from build123d import *

# Parameters (mm, degrees)
SCHIZZO1_W                   = 42.3
SCHIZZO1_H                   = 42.3
ESTRUSIONE_ESTRUSIONE1_DEPTH = 48
SMUSSO1_SIZE                 = 5
SCHIZZO2_R                   = 2.5
ESTRUSIONE_ESTRUSIONE2_DEPTH = 26
SCHIZZO3_W                   = 2.3
SCHIZZO3_H                   = 15
ESTRUSIONE_ESTRUSIONE3_DEPTH = 5
SCHIZZO4_R                   = 1.5
TAGLIO_ESTRUSIONE1_DEPTH     = 5


with BuildPart() as part:
    # Schizzo1 → Estrusione-Estrusione1 (new body)
    with BuildSketch(Plane.XY):
        Rectangle(SCHIZZO1_W, SCHIZZO1_H)
    extrude(amount=ESTRUSIONE_ESTRUSIONE1_DEPTH)

    # Smusso1
    smusso1_edges = [part.edges().sort_by_distance(p)[0] for p in [
        (21.15, -21.15, 24),
        (-21.15, -21.15, 24),
        (-21.15, 21.15, 24),
        (21.15, 21.15, 24),
    ]]
    chamfer(smusso1_edges, length=SMUSSO1_SIZE)

    # Schizzo2 → Estrusione-Estrusione2 (add)
    with BuildSketch(Plane.XY.offset(48)):
        Circle(SCHIZZO2_R)
    extrude(amount=ESTRUSIONE_ESTRUSIONE2_DEPTH)

    # Schizzo3 → Estrusione-Estrusione3 (add)
    with BuildSketch(Plane(origin=(0, 0, 0), x_dir=(-1, 0, 0), z_dir=(0, 0, -1))):
        with Locations((0, -28.65)):
            Rectangle(SCHIZZO3_W, SCHIZZO3_H)
    extrude(amount=-ESTRUSIONE_ESTRUSIONE3_DEPTH)

    # Schizzo4 → Taglio-Estrusione1 (cut)
    with BuildSketch(Plane.XY.offset(48)):
        with Locations((-15.5, 15.5)):
            Circle(SCHIZZO4_R)
        with Locations((-15.5, -15.5)):
            Circle(SCHIZZO4_R)
        with Locations((15.5, -15.5)):
            Circle(SCHIZZO4_R)
        with Locations((15.5, 15.5)):
            Circle(SCHIZZO4_R)
    extrude(amount=-TAGLIO_ESTRUSIONE1_DEPTH, mode=Mode.SUBTRACT)


solid = part.part
Verification items for the finished model (mm, model axes). A direction names the side the tool comes from. Give positions to 0.01 mm unless a question says otherwise; leave off trailing zeros. Loops run counter-clockwise (first coordinate to the right, second up) from the corner with the lowest first, then second, coordinate; pieces in that order, holes last.
1) Depth check by flat-ended pin: pin 1 Ø12 at (x, y) = (-2.5, 1) entering from -Z; pin 2 Ø3 at (y, z) = (3, 52) entering from -X; pin 3 Ø12 at (x, y) = (9.5, -12) entering from +Z; pin 4 Ø1.2 at (x, y) = (0, -25.5) entering from +Z. Enter the tip coordinate at first touch or a pass-through.
2) Thickness scan on line 1 along Y through (x, z) = (-15.5, 45); line 2 along X through (y, z) = (-15, 44). Record the ranges inside material, lowest first.
3) Draft check along Y on faces 1 (the flat face through (15, 16, 43)), 2 (the flat face through (-18.6, -18.7, 23.7)), 3 (the cylindrical face through (-0.54, -2.44, 60.82)). Enter one of: pulls with the +Y half, pulls with the -Y half, needs draft (parallel to the pull), parting line crosses it, or undercut.
4) Sectioned sample at C-C, the plane x = 0. Enter the section's corners in (y, z), then the cut area to 3 significant figures.
5) Set-up check for faces 4 (the flat face through (21.15, 0, 24)), 5 (the flat face through (0, -29, 5)), 6 (the flat face through (-16, 16, 43)), 7 (the flat face through (0, 21.15, 24)), 8 (the flat face through (1.15, -29, 2)): record each of +Z, -Z, +X, -X, +Y, -Y from which the full face is reachable in a straight line by a thin tool's end or side.
6) Sectioned sample at D-D, the plane y = 11.5. Enter the section's corners in (x, z).
7) Sectioned sample at B-B, the plane z = 26. Enter the section's corners in (x, y), then the cut area to 3 significant figures.
8) Sectioned sample at A-A, the plane y = 0. Enter the section's corners in (x, z), then the cut area to 3 significant figures.
Answers:
1. pin 1: stops at z = 0
1. pin 2: stops at x = -2
1. pin 3: stops at z = 48
1. pin 4: stops at z = 5
2. line 1: y = -21.15 to -17, -14 to 14, 17 to 21.15
2. line 2: x = -21.15 to -16.91, -14.09 to 14.09, 16.91 to 21.15
3. face 1: undercut
3. face 2: pulls with the -Y half
3. face 3: parting line crosses it
4. outline: (-36.15, 0) - (21.15, 0) - (21.15, 48) - (2.5, 48) - (2.5, 74) - (-2.5, 74) - (-2.5, 48) - (-21.15, 48) - (-21.15, 5) - (-36.15, 5) - close
4. area: 2,240 mm2
5. face 4: +Z, -Z, +X, +Y, -Y
5. face 5: +Z, +X, -X, -Y
5. face 6: +Z
5. face 7: +Z, -Z, +X, -X, +Y
5. face 8: +Z, -Z, +X, -Y
6. outline: (-21.15, 0) - (21.15, 0) - (21.15, 48) - (-21.15, 48) - close
7. outline: (-21.15, -16.15) - (-16.15, -21.15) - (16.15, -21.15) - (21.15, -16.15) - (21.15, 16.15) - (16.15, 21.15) - (-16.15, 21.15) - (-21.15, 16.15) - close
7. area: 1,740 mm2
8. outline: (-21.15, 0) - (21.15, 0) - (21.15, 48) - (2.5, 48) - (2.5, 74) - (-2.5, 74) - (-2.5, 48) - (-21.15, 48) - close
8. area: 2,160 mm2
